from build123d import *

# Parameters (mm, degrees)
F1_DEPTH = 66.548


with BuildPart() as f1:
    # F0 (on Right) → F1 (new body)
    with BuildSketch(Plane.YZ):
        Polygon((0, -5.588), (0, 5.588), (-58.913485, 5.588), (-58.913485, 29.855885), (-81.265485, 29.855885), (-81.265485, 5.588), (-81.265485, -5.588), (-58.913485, -5.588), align=None)
        Polygon((100.061485, 5.588), (58.913485, 5.588), (0, 5.588), (0, -5.588), (58.913485, -5.588), (58.913485, -17.083315), (100.061485, -17.083315), align=None)
    extrude(amount=-F1_DEPTH)


solid = f1.part
Design review of the part built by this model. Coordinates are the model's own, in mm. A direction names the side the tool comes from. Give positions to 0.01 mm unless a question says otherwise; leave off trailing zeros. Loops run counter-clockwise (first coordinate to the right, second up) from the corner with the lowest first, then second, coordinate; pieces in that order, holes last. Notation, with made-up numbers: (85.5, 29) -> (103.5, 29) arc R10 cw to (103.5, 48) -> close; hole circle Ø9 at (26.25, 31). An arc over 180 degrees is marked (long way). One line per question, with ' | ' between items. Start each with the question number.
(1) We need section B-B (z = 25). State the section outline as (x, y) points.
(2) Insertion check: P1, Ø4, axis at x = -45, y = -26.5, coming from the -Z side; P2, Ø12, axis at y = 14.5, z = 16, coming from the +X side; P3, Ø20, axis at x = -36.5, y = 30.5, coming from the +Z side. Each pin has a flat end and moves straight along its axis. Give the tip position at first contact, or say it passes through.
(3) For faces 1 (the face through (-33, 58.913, -11)), 2 (the face through (-33, 22, 5.588)), 3 (the face through (0, 9, 1)), list the 3-axis set-ups (+Z, -Z, +X, -X, +Y, -Y) from which the entire face can be reached by the end or side of a thin tool; tool diameter is ignored.
(4) We need section C-C (y = -9). State the section outline as (x, z) points.
(5) For line 1 (Z direction, x = -63, y = 82); line 2 (Y direction, x = -55.5, z = 17.5); line 3 (Z direction, x = -23, y = -19.5), list the stretches that pass through material, from the lowest coordinate up.
(6) We need section A-A (x = -51.5). State the section outline as (y, z) points.
The answers:
1) outline: (-66.55, -81.27) -> (0, -81.27) -> (0, -58.91) -> (-66.55, -58.91) -> close
2) P1: stops at z = -5.59 | P2: passes through | P3: stops at z = 5.59
3) face 1: -Z, +X, -X, -Y | face 2: +Z, +X, -X, +Y | face 3: +Z, -Z, +X, +Y, -Y
4) outline: (-66.55, -5.59) -> (0, -5.59) -> (0, 5.59) -> (-66.55, 5.59) -> close
5) line 1: z = -17.08 to 5.59 | line 2: y = -81.27 to -58.91 | line 3: z = -5.59 to 5.59
6) outline: (-81.27, -5.59) -> (58.91, -5.59) -> (58.91, -17.08) -> (100.06, -17.08) -> (100.06, 5.59) -> (-58.91, 5.59) -> (-58.91, 29.86) -> (-81.27, 29.86) -> close
